CAD build for the part. Positions are in the model's coordinates, mm. Give positions to 0.01 mm unless a question says otherwise; leave off trailing zeros. Order: outer loops, then holes, each group sorted by start corner. A loop starts at its lowest first (then second) coordinate and runs counter-clockwise, first axis right, second up.
Item 1: Band-saw the part on D-D on x = 31. Give the cut face in (y, z), plus the area to 3 significant figures.
Item 2: Band-saw the part on A-A on z = -27. Give the cut face in (x, y), plus the area to 3 significant figures.
Item 3: Flat gauge pin, fed straight in: P1, Ø1.5, axis at x = 9, y = 1.5, coming from the -Z side. Where does the tip first touch, or does it go through?
Item 4: Wall check: L1, parallel to X at y = 0.7, z = -10; L2, parallel to X at y = 0.95, z = -20.5 (3 decimals); L3, parallel to Z at x = 17, y = 0.4. Give the ranges that are in metal, low to high.
Item 5: Band-saw the part on C-C on x = 7.5. Give the cut face in (y, z) (3 decimals), plus the area to 4 significant figures.
Item 6: Band-saw the part on B-B on z = -101.5. Give the cut face in (x, y).
```python
from build123d import *

# Parameters (mm, degrees)
CROQUIS1_R              = 1.5
CROQUIS1_R_2            = 1.375
CROQUIS1_W              = 6.357227068
CROQUIS1_H              = 13.910539406
CROQUIS1_W_2            = 6.149922685
CROQUIS1_H_2            = 14.93552652
SALIENTE_EXTRUIR1_DEPTH = 3


with BuildPart() as part:
    # Croquis1 → Saliente-Extruir1 (new body)
    with BuildSketch(Plane(origin=(0, 0, 0), x_dir=(1, 0, 0), z_dir=(0, 1, 0))):
        Polygon((0, 0), (25, 0), (25, 3), (35, 3), (35, 0), (60, 0), (60, 57.5), (55, 57.5), (55, 67.5), (60, 67.5), (60, 125), (57.5, 125), (57.5, 122), (47.5, 122), (47.5, 125), (12.5, 125), (12.5, 122), (2.5, 122), (2.5, 125), (0, 125), (0, 67.5), (5, 67.5), (5, 57.5), (0, 57.5), align=None)
        with Locations(Location((20, 101.5, 0), (0, 0, 270))):
            Circle(CROQUIS1_R, mode=Mode.SUBTRACT)
        with Locations(Location((20, 121.5, 0), (0, 0, 270))):
            Circle(CROQUIS1_R, mode=Mode.SUBTRACT)
        with Locations(Location((40, 121.5, 0), (0, 0, 270))):
            Circle(CROQUIS1_R, mode=Mode.SUBTRACT)
        with Locations(Location((40, 101.5, 0), (0, 0, 270))):
            Circle(CROQUIS1_R, mode=Mode.SUBTRACT)
        with Locations(Location((7.5, 3, 0), (0, 0, 270))):
            Circle(CROQUIS1_R_2, mode=Mode.SUBTRACT)
        with Locations(Location((7.5, 20.5, 0), (0, 0, 270))):
            Circle(CROQUIS1_R_2, mode=Mode.SUBTRACT)
        with Locations(Location((56, 20.5, 0), (0, 0, 270))):
            Circle(CROQUIS1_R_2, mode=Mode.SUBTRACT)
        with Locations(Location((56, 3, 0), (0, 0, 270))):
            Circle(CROQUIS1_R_2, mode=Mode.SUBTRACT)
        with Locations((16.821386466, 11.689804861)):
            Rectangle(CROQUIS1_W, CROQUIS1_H, mode=Mode.SUBTRACT)
        with Locations((46.033519219, 11.689804861)):
            Rectangle(CROQUIS1_W_2, CROQUIS1_H_2, mode=Mode.SUBTRACT)
        with BuildLine():
            Line((10.5, 33.818022813), (10.5, 86.818022813))
            ThreePointArc((10.5, 86.818022813), (11.085786438, 88.232236376), (12.5, 88.818022813))
            Line((12.5, 88.818022813), (47.5, 88.818022813))
            ThreePointArc((47.5, 88.818022813), (48.914213562, 88.232236376), (49.5, 86.818022813))
            Line((49.5, 86.818022813), (49.5, 33.818022813))
            ThreePointArc((49.5, 33.818022813), (48.914213562, 32.403809251), (47.5, 31.818022813))
            ThreePointArc((47.5, 31.818022813), (46.085786438, 31.232236376), (45.5, 29.818022813))
            Line((45.5, 29.818022813), (45.5, 25.818022813))
            ThreePointArc((45.5, 25.818022813), (44.914213562, 24.403809251), (43.5, 23.818022813))
            Line((43.5, 23.818022813), (38.5, 23.818022813))
            ThreePointArc((38.5, 23.818022813), (37.085786438, 23.232236376), (36.5, 21.818022813))
            Line((36.5, 21.818022813), (36.5, 8.818022813))
            ThreePointArc((36.5, 8.818022813), (35.914213562, 7.403809251), (34.5, 6.818022813))
            Line((34.5, 6.818022813), (25.5, 6.818022813))
            ThreePointArc((25.5, 6.818022813), (24.085786438, 7.403809251), (23.5, 8.818022813))
            Line((23.5, 8.818022813), (23.5, 21.818022813))
            ThreePointArc((23.5, 21.818022813), (22.914213562, 23.232236376), (21.5, 23.818022813))
            Line((21.5, 23.818022813), (16.5, 23.818022813))
            ThreePointArc((16.5, 23.818022813), (15.085786438, 24.403809251), (14.5, 25.818022813))
            Line((14.5, 25.818022813), (14.5, 29.818022813))
            ThreePointArc((14.5, 29.818022813), (13.914213562, 31.232236376), (12.5, 31.818022813))
            ThreePointArc((12.5, 31.818022813), (11.085786438, 32.403809251), (10.5, 33.818022813))
        make_face(mode=Mode.SUBTRACT)
    extrude(amount=SALIENTE_EXTRUIR1_DEPTH)


solid = part.part
```
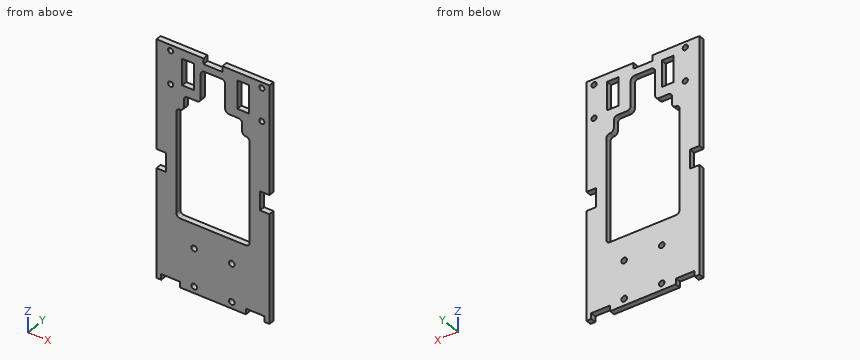
The answers:
1. outline: (0, -125) - (3, -125) - (3, -88.82) - (0, -88.82) - close; (0, -6.82) - (3, -6.82) - (3, -3) - (0, -3) - close
1. area: 120 mm2
2. outline: (0, 0) - (14.5, 0) - (14.5, 3) - (0, 3) - close; (45.5, 0) - (60, 0) - (60, 3) - (45.5, 3) - close
2. area: 87.0 mm2
3. P1: stops at z = -122
4. L1: x = 0 to 13.64, 20 to 23.5, 36.5 to 42.96, 49.11 to 60
4. L2: x = 0 to 6.125, 8.875 to 23.5, 36.5 to 54.625, 57.375 to 60
4. L3: z = -125 to -88.82, -23.82 to -18.65, -4.73 to 0
5. outline: (0, -122) - (3, -122) - (3, -21.875) - (0, -21.875) - close; (0, -19.125) - (3, -19.125) - (3, -4.375) - (0, -4.375) - close; (0, -1.625) - (3, -1.625) - (3, 0) - (0, 0) - close
5. area: 349.5 mm2
6. outline: (0, 0) - (18.5, 0) - (18.5, 3) - (0, 3) - close; (21.5, 0) - (38.5, 0) - (38.5, 3) - (21.5, 3) - close; (41.5, 0) - (60, 0) - (60, 3) - (41.5, 3) - close
